Design review of the part built by this model. Coordinates are the model's own, in mm. A direction names the side the tool comes from. Give positions to 0.01 mm unless a question says otherwise; leave off trailing zeros. Write each loop counter-clockwise with the first axis right and the second up, starting at its lowest first coordinate (ties: lowest second). Pieces come first, ordered by that corner, then holes.
Autodesk Fusion 360 part; units mm, degrees
sketch "스케치1" plane through (0, 0, 0) normal (0, 0, 1) x (1, 0, 0)
  line L0 (0, 0) -> (60, 0)
  line L1 (60, 0) -> (60, 30)
  line L2 (60, 30) -> (0, 30)
  line L3 (0, 30) -> (0, 0)
  dimension "d1" = 60
  dimension "d2" = 30
extrude "돌출1" add sketch "스케치1" along normal blind 2
sketch "스케치5" plane through (0, 0, 2) normal (0, 0, 1) x (-1, 0, 0)
  line L0 (0, -30) -> (0, 0)
  line L1 (0, 0) -> (0, -30)
  line L2 (-60, -30) -> (0, -30)
  line L3 (-60, -30) -> (-60, 0)
  line L4 (0, 0) -> (-60, 0)
  line L5 (-60, 0) -> (-54, 0)
  line L6 (-54, -28) -> (-6, -28)
  line L7 (-2, -24) -> (-2, -6)
  line L8 (-6, 0) -> (0, 0)
  line L9 (-58, -24) -> (-58, -6)
  line L10 (-2, -24) -> (-6, -24)
  line L11 (-6, -24) -> (-6, -28)
  line L12 (-54, -28) -> (-54, -24)
  line L13 (-54, -24) -> (-58, -24)
  line L14 (-2, -6) -> (-6, -6)
  line L15 (0, 0) -> (-60, 0)
  line L16 (-6, -6) -> (-6, 0)
  line L17 (-58, -6) -> (-54, -6)
  line L18 (-54, -6) -> (-54, 0)
  point P0 (0, -30)
  point P1 (-60, -30)
  point P2 (-60, 0)
  dimension "d38" = 2
  dimension "d39" = 2
  dimension "d42" = 2
  dimension "d43" = 6
  dimension "d44" = 6
  dimension "d45" = 6
  dimension "d46" = 6
  dimension "d47" = 6
extrude "돌출11" add sketch "스케치5" along normal blind 2 contours L0 L1 L2 L3 L4 L5 L6 L7 L8 L9 L10 L11 L12 L13 L14 L15 L16 L17 L18
sketch "스케치10" plane through (0, 0, 4) normal (0, 0, 1) x (-1, 0, 0)
  circle A0 centre (-57, -3) radius 1
  circle A1 centre (-57, -27) radius 1
  circle A2 centre (-3, -3) radius 1
  circle A3 centre (-3, -27) radius 1
  dimension "d82" = 2
  dimension "d83" = 3
  dimension "d84" = 3
  dimension "d85" = 24
  dimension "d86" = 54
extrude "돌출13" cut sketch "스케치10" against normal blind 4
fillet "필렛4" radius 3 10 edges at (0, 0, 2) (60, 0, 2) (0, 30, 2) (60, 30, 2) (54, 24, 3) (6, 24, 3) (6, 6, 3) (54, 6, 3) (6, 0, 3) (54, 0, 3)
chamfer "챔퍼1" distance 1.5 angle 45 4 edges at (57.9323, 3.3616, 0) (57.9323, 27.3616, 0) (3.9323, 27.3616, 0) (3.9323, 3.3616, 0)
sketch "스케치11" plane through (0, 0, 2) normal (0, 0, 1) x (-1, 0, 0)
  circle A0 centre (-45, -8.1) radius 2.3
  circle A1 centre (-15, -8.1) radius 2.3
  dimension "d93" = 8.1
  dimension "d95" = 4.6
  dimension "d98" = 15
  dimension "d99" = 30
extrude "돌출14" add sketch "스케치11" along normal blind 1.5
(1) Consider section C-C, the plane x = 15. Give the boundary of the cut face in (y, z), then the cut area to 3 significant figures.
Resolved:
outline: (0, 0) - (30, 0) - (30, 4) - (28, 4) - (28, 2) - (10.4, 2) - (10.4, 3.5) - (5.8, 3.5) - (5.8, 2) - (0, 2) - close
area: 70.9 mm2
(2) Clearance check with flat-ended pins moving along their axes: P1, Ø14, axis at x = 44, y = 8.5, coming from the +Z side; P2, Ø0.6, axis at x = 40.5, z = 2.5, coming from the -Y side; P3, Ø0.5, axis at x = 57.5, z = 3.5, coming from the -Y side. State where each tip first meets the part, or that it passes through.
Resolved:
P1: stops at z = 3.5
P2: stops at y = 28
P3: stops at y = 0.01
(3) Tool access review of faces 1 (the face through (54.86, 0.9, 3.01)), 2 (the face through (58, 15, 3)), 3 (the face through (0.86, 29.1, 1.97)): name each direction out of +Z, -Z, +X, -X, +Y, -Y from which nothing blocks a thin tool from reaching the whole face with its end or side.
Resolved:
face 1: +Z, -Y
face 2: +Z
face 3: +Z, -Z, -X, +Y
(4) Consider section D-D, the plane y = 22.75. Give the boundary of the cut face in (x, z), then the cut area to 3 significant figures.
Resolved:
outline: (0, 0) - (60, 0) - (60, 4) - (58, 4) - (58, 2) - (2, 2) - (2, 4) - (0, 4) - close
area: 128 mm2
(5) To check wall thickness, follow L1, parallel to X at y = 3, z = 2.25; L2, parallel to X at y = 8, z = 3; L3, parallel to Y at x = 3, z = 3.3. State the ranges of each line that lie inside material, in increasing order.
Resolved:
L1: x = 0 to 2, 4 to 6, 54 to 56, 58 to 60
L2: x = 0 to 2, 12.7 to 17.3, 42.7 to 47.3, 58 to 60
L3: y = 0 to 2, 4 to 6, 24 to 26, 28 to 30
(6) Consider section A-A, the plane z = 0.8. Give the boundary of the cut face in (x, y), then the cut area to 3 significant figures.
Resolved:
outline: (0, 3) arc R3 ccw to (3, 0) - (57, 0) arc R3 ccw to (60, 3) - (60, 27) arc R3 ccw to (57, 30) - (3, 30) arc R3 ccw to (0, 27) - close; hole circle Ø3.4 at (3, 3); hole circle Ø3.4 at (3, 27); hole circle Ø3.4 at (57, 3); hole circle Ø3.4 at (57, 27)
area: 1,760 mm2
(7) Mouldability with a two-part tool opening along X and no side actions: class faces 4 (the face through (30, 0, 1)), 5 (the face through (3.737, 26.324, 2.768)), 6 (the face through (59.1, 0.86, 2.03)) as pulls with the +X half, pulls with the -X half, needs draft (parallel to the pull), parting line crosses it, or undercut.
Resolved:
face 4: needs draft
face 5: undercut
face 6: pulls with the +X half
(8) Consider section B-B, the plane y = 8.1. Give the boundary of the cut face in (x, z).
Resolved:
outline: (0, 0) - (60, 0) - (60, 4) - (58, 4) - (58, 2) - (47.3, 2) - (47.3, 3.5) - (42.7, 3.5) - (42.7, 2) - (17.3, 2) - (17.3, 3.5) - (12.7, 3.5) - (12.7, 2) - (2, 2) - (2, 4) - (0, 4) - close
